```python
from build123d import *

# Parameters (mm, degrees)
SKETCH1_W           = 40
SKETCH1_H           = 62
BOSS_EXTRUDE1_DEPTH = 12


# Read off the part's stored shape, not the designer's step: AdvancedHole1
with BuildPart() as part:
    # Sketch1 → Boss-Extrude1 (new body)
    with BuildSketch(Plane(origin=(0, 0, 0), x_dir=(1, 0, 0), z_dir=(0, 1, 0))):
        Rectangle(SKETCH1_W, SKETCH1_H)
    extrude(amount=BOSS_EXTRUDE1_DEPTH)

    # AdvancedHole1 outline → AdvancedHole1 (revolve, cut)
    with BuildSketch(Plane.XY.offset(-19)):
        Polygon((4.5, 4.46), (4.5, 12), (0, 12), (0, 0), (8.96, 0), align=None)
    revolve(axis=Axis((0, 0, -19), (0, 1, 0)), mode=Mode.SUBTRACT)

    # AdvancedHole1 2 outline → AdvancedHole1 2 (revolve, cut)
    with BuildSketch(Plane.XY.offset(19)):
        Polygon((4.5, 4.46), (4.5, 12), (0, 12), (0, 0), (8.96, 0), align=None)
    revolve(axis=Axis((0, 0, 19), (0, 1, 0)), mode=Mode.SUBTRACT)


solid = part.part
```
Part model, mm, in its own coordinate system. Round coordinates to 2 decimals unless told otherwise and drop trailing zeros. Loops run counter-clockwise (first coordinate to the right, second up) from the corner with the lowest first, then second, coordinate; pieces in that order, holes last.
Item 1: Drop flat-ended pins along their axis: P1, Ø10.5, axis at x = 0, z = 19, coming from the -Y side; P2, Ø5.5, axis at x = 0, z = -19, coming from the -Y side. Give the stop position or say it passes through.
Item 2: Cut at A-A, the plane z = 19. Give the cut face in (x, y).
Item 3: Mould opens along X. For faces 1 (the face through (0, 0, 0)), 2 (the face through (20, 6, 0)), 3 (the face through (-0.61, 4.24, 14.32)) say: +X half, -X half, draft (parallel to the pull), parting line (faces both ways), or undercut.
Item 4: Drill centre lines: line 1 (Z direction, x = 0, y = 8); line 2 (X direction, y = 7, z = 19); line 3 (Z direction, x = -2.5, y = 5.5). Where is each one in solid material? Low to high.
Item 5: Cut at D-D, the plane y = 7.5. Give the cut face in (x, z), then the cut area to 3 significant figures.
Item 6: Cut at C-C, the plane y = 3. Give the cut face in (x, z).
Item 7: Cut at B-B, the plane x = 0. Give the cut face in (y, z).
A:
1. P1: stops at y = 3.71
1. P2: passes through
2. outline: (-20, 0) - (-8.96, 0) - (-4.5, 4.46) - (-4.5, 12) - (-20, 12) - close; (4.5, 4.46) - (8.96, 0) - (20, 0) - (20, 12) - (4.5, 12) - close
3. face 1: draft
3. face 2: +X half
3. face 3: undercut
4. line 1: z = -31 to -23.5, -14.5 to 14.5, 23.5 to 31
4. line 2: x = -20 to -4.5, 4.5 to 20
4. line 3: z = -31 to -22.74, -15.26 to 15.26, 22.74 to 31
5. outline: (-20, -31) - (20, -31) - (20, 31) - (-20, 31) - close; hole circle Ø9 at (0, -19); hole circle Ø9 at (0, 19)
5. area: 2,350 mm2
6. outline: (-20, -31) - (20, -31) - (20, 31) - (-20, 31) - close; hole circle Ø11.92 at (0, -19); hole circle Ø11.92 at (0, 19)
7. outline: (0, -31) - (12, -31) - (12, -23.5) - (4.46, -23.5) - (0, -27.96) - close; (0, -10.04) - (4.46, -14.5) - (12, -14.5) - (12, 14.5) - (4.46, 14.5) - (0, 10.04) - close; (0, 27.96) - (4.46, 23.5) - (12, 23.5) - (12, 31) - (0, 31) - close
